```python
from build123d import *

# Parameters (mm, degrees)
F0_W     = 482.6
F0_H     = 177.8
F1_DEPTH = 1.56
F2_R     = 2.5
F3_R     = 2.55
F4_DEPTH = 25


with BuildPart() as f1:
    # F0 (on Top) → F1 (new body)
    with BuildSketch(Plane.XY):
        with Locations((241.3, 88.9)):
            Rectangle(F0_W, F0_H)
        with BuildLine():
            Line((7, 41.4), (10.76, 41.4))
            ThreePointArc((10.76, 41.4), (13.022742, 40.462742), (13.96, 38.2))
            Line((13.96, 38.2), (13.96, 38))
            ThreePointArc((13.96, 38), (13.022742, 35.737258), (10.76, 34.8))
            Line((10.76, 34.8), (7, 34.8))
            ThreePointArc((7, 34.8), (4.737258, 35.737258), (3.8, 38))
            Line((3.8, 38), (3.8, 38.2))
            ThreePointArc((3.8, 38.2), (4.737258, 40.462742), (7, 41.4))
        make_face(mode=Mode.SUBTRACT)
        with BuildLine():
            Line((468.64, 38), (468.64, 38.2))
            ThreePointArc((468.64, 38.2), (469.577258, 40.462742), (471.84, 41.4))
            Line((471.84, 41.4), (475.6, 41.4))
            ThreePointArc((475.6, 41.4), (477.862742, 40.462742), (478.8, 38.2))
            Line((478.8, 38.2), (478.8, 38))
            ThreePointArc((478.8, 38), (477.862742, 35.737258), (475.6, 34.8))
            Line((475.6, 34.8), (471.84, 34.8))
            ThreePointArc((471.84, 34.8), (469.577258, 35.737258), (468.64, 38))
        make_face(mode=Mode.SUBTRACT)
        with BuildLine():
            Line((10.76, 136.4), (7, 136.4))
            ThreePointArc((7, 136.4), (4.737258, 137.337258), (3.8, 139.6))
            Line((3.8, 139.6), (3.8, 139.8))
            ThreePointArc((3.8, 139.8), (4.737258, 142.062742), (7, 143))
            Line((7, 143), (10.76, 143))
            ThreePointArc((10.76, 143), (13.022742, 142.062742), (13.96, 139.8))
            Line((13.96, 139.8), (13.96, 139.6))
            ThreePointArc((13.96, 139.6), (13.022742, 137.337258), (10.76, 136.4))
        make_face(mode=Mode.SUBTRACT)
        with BuildLine():
            Line((478.8, 139.8), (478.8, 139.6))
            ThreePointArc((478.8, 139.6), (477.862742, 137.337258), (475.6, 136.4))
            Line((475.6, 136.4), (471.84, 136.4))
            ThreePointArc((471.84, 136.4), (469.577258, 137.337258), (468.64, 139.6))
            Line((468.64, 139.6), (468.64, 139.8))
            ThreePointArc((468.64, 139.8), (469.577258, 142.062742), (471.84, 143))
            Line((471.84, 143), (475.6, 143))
            ThreePointArc((475.6, 143), (477.862742, 142.062742), (478.8, 139.8))
        make_face(mode=Mode.SUBTRACT)
    extrude(amount=F1_DEPTH)

    # F2
    f2_edges = [f1.edges().sort_by_distance(p)[0] for p in [
        (0, 177.8, 0.78),
        (0, 0, 0.78),
        (482.6, 177.8, 0.78),
        (482.6, 0, 0.78),
    ]]
    fillet(f2_edges, radius=F2_R)

    # F3 (on face) → F4 (cut)
    with BuildSketch(Plane.XY.offset(1.56)):
        with BuildLine():
            Line((136.768348, 147.55), (103.231652, 147.55))
            ThreePointArc((103.231652, 147.55), (76.866486, 132.033514), (61.35, 105.668348))
            Line((61.35, 105.668348), (61.35, 72.131652))
            ThreePointArc((61.35, 72.131652), (76.866486, 45.766486), (103.231652, 30.25))
            Line((103.231652, 30.25), (136.768348, 30.25))
            ThreePointArc((136.768348, 30.25), (163.133514, 45.766486), (178.65, 72.131652))
            Line((178.65, 72.131652), (178.65, 105.668348))
            ThreePointArc((178.65, 105.668348), (163.133514, 132.033514), (136.768348, 147.55))
        make_face()
        with Locations((67.55, 141.35)):
            Circle(F3_R)
        with Locations((67.55, 36.45)):
            Circle(F3_R)
        with Locations((172.45, 141.35)):
            Circle(F3_R)
        with Locations((172.45, 36.45)):
            Circle(F3_R)
        with BuildLine():
            Line((379.368348, 147.55), (345.831652, 147.55))
            ThreePointArc((345.831652, 147.55), (319.466486, 132.033514), (303.95, 105.668348))
            Line((303.95, 105.668348), (303.95, 72.131652))
            ThreePointArc((303.95, 72.131652), (319.466486, 45.766486), (345.831652, 30.25))
            Line((345.831652, 30.25), (379.368348, 30.25))
            ThreePointArc((379.368348, 30.25), (405.733514, 45.766486), (421.25, 72.131652))
            Line((421.25, 72.131652), (421.25, 105.668348))
            ThreePointArc((421.25, 105.668348), (405.733514, 132.033514), (379.368348, 147.55))
        make_face()
        with Locations((415.05, 36.45)):
            Circle(F3_R)
        with Locations((310.15, 36.45)):
            Circle(F3_R)
        with Locations((415.05, 141.35)):
            Circle(F3_R)
        with Locations((310.15, 141.35)):
            Circle(F3_R)
        with BuildLine():
            Line((239.8, 103.275), (239.8, 102.567937))
            ThreePointArc((239.8, 102.567937), (241.3, 75.15), (242.8, 102.567937))
            Line((242.8, 102.567937), (242.8, 103.275))
            Line((242.8, 103.275), (241.3, 103.275))
            Line((241.3, 103.275), (239.8, 103.275))
        make_face()
    extrude(amount=-F4_DEPTH, mode=Mode.SUBTRACT)


solid = f1.part
```
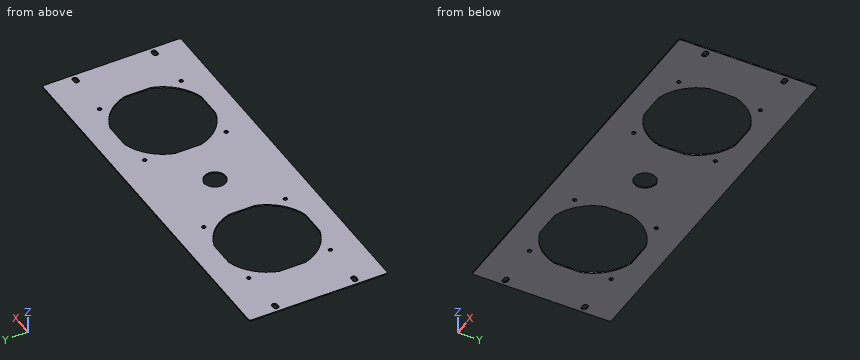
For this review, take the finished solid that the model builds, in its own axes (mm). Coordinates: 2 decimals unless noted, no trailing zeros. Loops run counter-clockwise (first coordinate to the right, second up) from the corner with the lowest first, then second, coordinate; pieces in that order, holes last. Notation, with made-up numbers: (-38.75, -35.5) - (-6.75, -35.5) arc R27 ccw to (-6.75, -12.5) - close; hole circle Ø10 at (42.25, 2). An arc over 180 degrees is marked (long way). Use one line per item in the form item = value. Start each with the question number.
1) Take a section at B-B (x = 350). State the section outline as (y, z) points.
2) Take a section at C-C (y = 65.5). State the section outline as (x, z) points, plus the area to 3 significant figures.
3) Take a section at A-A (y = 88.9). State the section outline as (x, z) points, plus the area to 3 significant figures.
4) For pin 1 (4 mm diameter, centred on x = 172.45, y = 36.45, fed in from +Z), flat-tipped, find the tip position at first contact; note if it passes through.
5) To check wall thickness, follow probe 1 along X at (y, z) = (49.5, 1.1); probe 2 along Y at (x, z) = (310.15, 0.6); probe 3 along X at (y, z) = (88.9, 0.7). State the ranges of each line that lie inside material, in increasing order. Write a range as from..to.
6) Take a section at D-D (z = 1.05). State how many separate pieces and enclosed holes the cut face has, plus the area to 3 significant figures.
From the geometry:
q1.outline = (0, 0) - (30.25, 0) - (30.25, 1.56) - (0, 1.56) - close; (147.55, 0) - (177.8, 0) - (177.8, 1.56) - (147.55, 1.56) - close
q2.outline = (0, 0) - (63.67, 0) - (63.67, 1.56) - (0, 1.56) - close; (176.33, 0) - (306.27, 0) - (306.27, 1.56) - (176.33, 1.56) - close; (418.93, 0) - (482.6, 0) - (482.6, 1.56) - (418.93, 1.56) - close
q2.area = 401 mm2
q3.outline = (0, 0) - (61.35, 0) - (61.35, 1.56) - (0, 1.56) - close; (178.65, 0) - (227.55, 0) - (227.55, 1.56) - (178.65, 1.56) - close; (255.05, 0) - (303.95, 0) - (303.95, 1.56) - (255.05, 1.56) - close; (421.25, 0) - (482.6, 0) - (482.6, 1.56) - (421.25, 1.56) - close
q3.area = 344 mm2
q4.pin_1 = through
q5.probe_1 = 0..73.43, 166.57..316.03, 409.17..482.6
q5.probe_2 = 0..33.9, 39..57.76, 120.04..138.8, 143.9..177.8
q5.probe_3 = 0..61.35, 178.65..227.55, 255.05..303.95, 421.25..482.6
q6.separate_pieces = 1
q6.enclosed_holes = 15
q6.area = 61,900 mm2
